```python
from build123d import *

# Parameters (mm, degrees)
EXTRUDE_1_DEPTH     = 20
SKETCH_2_R          = 1.7
CUT_EXTRUDE_1_DEPTH = 41.620192023
FILLET_1_R          = 2
FILLET_2_R          = 2


with BuildPart() as part:
    # ｽｹｯﾁ1 → ﾎﾞｽ - 押し出し1 (new body)
    with BuildSketch(Plane.XY):
        Polygon((0, 0), (-35, 0), (-30, 5), (0, 5), align=None)
    extrude(amount=EXTRUDE_1_DEPTH)

    # ｽｹｯﾁ2 → ｶｯﾄ - 押し出し1 (cut, through all)
    with BuildSketch(Plane(origin=(0, 5, 0), x_dir=(1, 0, 0), z_dir=(0, 1, 0))):
        with Locations(Location((-2.5, -10, 0), (0, 0, 270))):
            Circle(SKETCH_2_R)
    extrude(amount=-CUT_EXTRUDE_1_DEPTH, mode=Mode.SUBTRACT)

    # ﾌｨﾚｯﾄ1
    fillet_1_edges = [part.edges().sort_by_distance(p)[0] for p in [
        (-15, 5, 0),
        (-30, 5, 10),
        (-15, 5, 20),
    ]]
    fillet(fillet_1_edges, radius=FILLET_1_R)

    # ﾌｨﾚｯﾄ2
    fillet_2_edges = [part.edges().sort_by_distance(p)[0] for p in [
        (-35, 0, 10),
    ]]
    fillet(fillet_2_edges, radius=FILLET_2_R)


solid = part.part
```
Read the model definition and answer for the solid it produces. Units are mm, in the model's axes. Give positions to 0.01 mm unless a question says otherwise; leave off trailing zeros. Write each loop counter-clockwise with the first axis right and the second up, starting at its lowest first coordinate (ties: lowest second). Pieces come first, ordered by that corner, then holes. Notation, with made-up numbers: (86, -7) -> (97, -7) arc R8 cw to (97, 5) -> close; hole circle Ø6 at (83.25, 6). An arc over 180 degrees is marked (long way). Answer in a Markdown table with one row per item.
1) Section B-B on z = 10 is taken. Give the vertices of the cut face in (x, y).
Results list:
| item | result |
|---|---|
| outline | (-31.59, 3.41) arc R2 ccw to (-30.17, 0) -> (-4.2, 0) -> (-4.2, 5) -> (-29.17, 5) arc R2 ccw to (-30.59, 4.41) -> close; (-0.8, 0) -> (0, 0) -> (0, 5) -> (-0.8, 5) -> close |
2) Straight lines are drawn through the part: line 1 (X direction, y = 0.75, z = 8.75); line 2 (Z direction, x = -30, y = 3.4); line 3 (X direction, y = 3.5, z = 10). For each, find the intervals that lie inside material, in ascending order. Write a range as [from, to].
Results list:
| item | result |
|---|---|
| line 1 | [-31.73, -3.65], [-1.35, 0] |
| line 2 | [0.04, 19.96] |
| line 3 | [-31.5, -4.2], [-0.8, 0] |
3) Section C-C on y = 0.95 is taken. Give the vertices of the cut face in (x, z), plus the area to 3 significant figures.
Results list:
| item | result |
|---|---|
| outline | (-31.87, 0) -> (0, 0) -> (0, 20) -> (-31.87, 20) -> close; hole circle Ø3.4 at (-2.5, 10) |
| area | 628 mm^2 |
4) Section D-D on z = 3.5 is taken. Give the vertices of the cut face in (x, y).
Results list:
| item | result |
|---|---|
| outline | (-31.59, 3.41) arc R2 ccw to (-30.17, 0) -> (0, 0) -> (0, 5) -> (-29.17, 5) arc R2 ccw to (-30.59, 4.41) -> close |
5) Determine the mould class of faces 1 (the flat face through (-16, 2, 20)), 2 (the flat face through (0, 3, 10)), 3 (the cylindrical face through (-1.99, 2.54, 11.62)) for opening direction Z: released by +Z, released by -Z, zero draft, split by the parting line, or undercut.
Results list:
| item | result |
|---|---|
| face 1 | released by +Z |
| face 2 | zero draft |
| face 3 | undercut |
6) Section A-A on x = -2.5 is taken. Give the vertices of the cut face in (y, z), plus the area to 3 significant figures.
Results list:
| item | result |
|---|---|
| outline | (0, 0) -> (3, 0) arc R2 ccw to (5, 2) -> (5, 8.3) -> (0, 8.3) -> close; (0, 11.7) -> (5, 11.7) -> (5, 18) arc R2 ccw to (3, 20) -> (0, 20) -> close |
| area | 81.3 mm^2 |
7) Each of these flat-tipped pins is pushed along its axis until it touches: pin 1 Ø4 at (x, z) = (-2.5, 10) entering from +Y; pin 2 Ø2 at (y, z) = (4, 16.5) entering from -X. Where does it stop, or does it pass through?
Results list:
| item | result |
|---|---|
| pin 1 | y = 5 |
| pin 2 | x = -31.9 |
